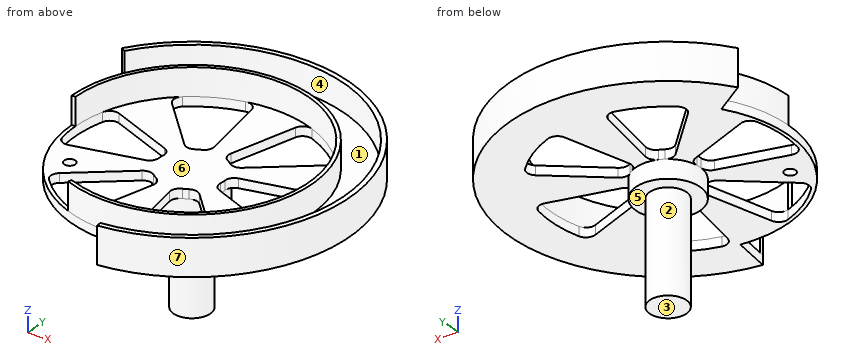
```python
from build123d import *
from build123d.topology import SkipClean

# Parameters (mm, degrees)
SCHIZZO2_R                   = 65.5
ESTRUSIONE_ESTRUSIONE1_DEPTH = 5
TAGLIO_ESTRUSIONE1_DEPTH     = 5
ESTRUSIONE_ESTRUSIONE2_START = 15
ESTRUSIONE_ESTRUSIONE2_DEPTH = 15
ESTRUSIONE_ESTRUSIONE3_DEPTH = 5
ESTRUSIONE_ESTRUSIONE4_DEPTH = 15
SCHIZZO7_R                   = 17.5
ESTRUSIONE_ESTRUSIONE5_DEPTH = 10
SCHIZZO8_R                   = 10
ESTRUSIONE_ESTRUSIONE6_DEPTH = 55
SCHIZZO9_R                   = 3
TAGLIO_ESTRUSIONE2_DEPTH     = 141.058619156


with BuildPart() as part:
    # Schizzo2 → Estrusione-Estrusione1 (new body)
    with BuildSketch(Plane.XY):
        Circle(SCHIZZO2_R)
    extrude(amount=ESTRUSIONE_ESTRUSIONE1_DEPTH)

    # Schizzo3 → Taglio-Estrusione1 (cut)
    with BuildSketch(Plane.XY.offset(5)):
        with BuildLine():
            ThreePointArc((-15.580303655, 61.558948481), (-11.6121535, 60.893291099), (-9.419229509, 57.519806288))
            Line((-9.419229509, 57.519806288), (-3.545169438, 21.649059417))
            ThreePointArc((-3.545169438, 21.649059417), (-4.118256573, 18.395634586), (-6.595126238, 16.20969802))
            ThreePointArc((-6.595126238, 16.20969802), (-7.944833745, 15.592614173), (-9.237403233, 14.863390647))
            ThreePointArc((-9.237403233, 14.863390647), (-12.461730523, 14.144422271), (-15.430658669, 15.593100175))
            Line((-15.430658669, 15.593100175), (-40.998016607, 41.429610598))
            ThreePointArc((-40.998016607, 41.429610598), (-42.438254768, 45.186607995), (-40.644362762, 48.788172498))
            ThreePointArc((-40.644362762, 48.788172498), (-28.828396733, 56.578914286), (-15.580303655, 61.558948481))
        make_face()
        with BuildLine():
            ThreePointArc((10.740447155, 13.816395873), (9.531183113, 14.676734939), (8.25337227, 15.431521188))
            ThreePointArc((8.25337227, 15.431521188), (6.018563747, 17.864386344), (5.788691541, 21.159892491))
            Line((5.788691541, 21.159892491), (15.380086943, 56.220129185))
            ThreePointArc((15.380086943, 56.220129185), (17.91362305, 59.345910719), (21.929615406, 59.593136921))
            ThreePointArc((21.929615406, 59.593136921), (34.584578723, 53.255581065), (45.521461387, 44.272413004))
            ThreePointArc((45.521461387, 44.272413004), (46.929060262, 40.503065473), (45.103998712, 36.917195183))
            Line((45.103998712, 36.917195183), (16.976050705, 13.894736502))
            ThreePointArc((16.976050705, 13.894736502), (13.871958583, 12.764332104), (10.740447155, 13.816395873))
        make_face()
        with BuildLine():
            ThreePointArc((17.335573392, -2.393302147), (17.476016858, -0.915879234), (17.490775503, 0.568130541))
            ThreePointArc((17.490775503, 0.568130541), (18.48029427, 3.719964073), (21.219350209, 5.566792317))
            Line((21.219350209, 5.566792317), (56.37810355, 14.790518587))
            ThreePointArc((56.37810355, 14.790518587), (60.351877818, 14.159302724), (62.573978168, 10.804964424))
            ThreePointArc((62.573978168, 10.804964424), (63.412975457, -3.323333221), (61.101765042, -17.286535477))
            ThreePointArc((61.101765042, -17.286535477), (58.541213762, -20.390225626), (54.523228221, -20.602611105))
            Line((54.523228221, -20.602611105), (20.521220142, -7.754322915))
            ThreePointArc((20.521220142, -7.754322915), (17.990215156, -5.631302481), (17.335573392, -2.393302147))
        make_face()
        with BuildLine():
            ThreePointArc((6.595126238, -16.20969802), (7.944833745, -15.592614173), (9.237403233, -14.863390647))
            ThreePointArc((9.237403233, -14.863390647), (12.461730523, -14.144422271), (15.430658669, -15.593100175))
            Line((15.430658669, -15.593100175), (40.998016607, -41.429610598))
            ThreePointArc((40.998016607, -41.429610598), (42.438254768, -45.186607995), (40.644362762, -48.788172498))
            ThreePointArc((40.644362762, -48.788172498), (28.828396733, -56.578914286), (15.580303655, -61.558948481))
            ThreePointArc((15.580303655, -61.558948481), (11.6121535, -60.893291099), (9.419229509, -57.519806288))
            Line((9.419229509, -57.519806288), (3.545169438, -21.649059417))
            ThreePointArc((3.545169438, -21.649059417), (4.118256573, -18.395634586), (6.595126238, -16.20969802))
        make_face()
        with BuildLine():
            ThreePointArc((-10.740447155, -13.816395873), (-9.531183113, -14.676734939), (-8.25337227, -15.431521188))
            ThreePointArc((-8.25337227, -15.431521188), (-6.018563747, -17.864386344), (-5.788691541, -21.159892491))
            Line((-5.788691541, -21.159892491), (-15.380086943, -56.220129185))
            ThreePointArc((-15.380086943, -56.220129185), (-17.91362305, -59.345910719), (-21.929615406, -59.593136921))
            ThreePointArc((-21.929615406, -59.593136921), (-34.584578723, -53.255581065), (-45.521461387, -44.272413004))
            ThreePointArc((-45.521461387, -44.272413004), (-46.929060262, -40.503065473), (-45.103998712, -36.917195183))
            Line((-45.103998712, -36.917195183), (-16.976050705, -13.894736502))
            ThreePointArc((-16.976050705, -13.894736502), (-13.871958583, -12.764332104), (-10.740447155, -13.816395873))
        make_face()
        with BuildLine():
            ThreePointArc((-17.335573392, 2.393302147), (-17.476016858, 0.915879234), (-17.490775503, -0.568130541))
            ThreePointArc((-17.490775503, -0.568130541), (-18.48029427, -3.719964073), (-21.219350209, -5.566792317))
            Line((-21.219350209, -5.566792317), (-56.37810355, -14.790518587))
            ThreePointArc((-56.37810355, -14.790518587), (-60.351877818, -14.159302724), (-62.573978168, -10.804964424))
            ThreePointArc((-62.573978168, -10.804964424), (-63.412975457, 3.323333221), (-61.101765042, 17.286535477))
            ThreePointArc((-61.101765042, 17.286535477), (-58.541213762, 20.390225626), (-54.523228221, 20.602611105))
            Line((-54.523228221, 20.602611105), (-20.521220142, 7.754322915))
            ThreePointArc((-20.521220142, 7.754322915), (-17.990215156, 5.631302481), (-17.335573392, 2.393302147))
        make_face()
    extrude(amount=-TAGLIO_ESTRUSIONE1_DEPTH, mode=Mode.SUBTRACT)

    # Schizzo4 → Estrusione-Estrusione2 (add)
    with SkipClean():  # the faces are left unmerged after this step: merging them gives an invalid solid
        with BuildSketch(Plane.XY.offset(5).offset(ESTRUSIONE_ESTRUSIONE2_START)):
            with BuildLine():
                Line((-65.499588659, 0.23213256), (-63.499601219, 0.225044543))
                ThreePointArc((-63.499601219, 0.225044543), (52.144908397, 36.23752928), (-21.929615406, -59.593136921))
                Line((-21.929615406, -59.593136921), (-22.620311954, -61.470086116))
                ThreePointArc((-22.620311954, -61.470086116), (53.787267716, 37.378868785), (-65.499588659, 0.23213256))
            make_face()
        extrude(amount=-ESTRUSIONE_ESTRUSIONE2_DEPTH)

    # Schizzo5 → Estrusione-Estrusione3 (add)
    with SkipClean():  # the faces are left unmerged after this step: merging them gives an invalid solid
        with BuildSketch(Plane.XY):
            with BuildLine():
                Line((-71.941161318, 46.719136424), (-54.9329222, 35.673856793))
                ThreePointArc((-54.9329222, 35.673856793), (55.547150298, 34.709711807), (7.982441993, -65.011772933))
                Line((7.982441993, -65.011772933), (10.453952277, -85.140608888))
                ThreePointArc((10.453952277, -85.140608888), (72.745565688, 45.456474486), (-71.941161318, 46.719136424))
            make_face()
        extrude(amount=ESTRUSIONE_ESTRUSIONE3_DEPTH)

    # Schizzo6 → Estrusione-Estrusione4 (add)
    with SkipClean():  # the faces are left unmerged after this step: merging them gives an invalid solid
        with BuildSketch(Plane.XY.offset(5)):
            with BuildLine():
                Line((-71.941161318, 46.719136424), (-69.71449096, 45.273119786))
                ThreePointArc((-69.71449096, 45.273119786), (70.493997993, 44.049538839), (10.130389171, -82.505398855))
                Line((10.130389171, -82.505398855), (10.453952277, -85.140608888))
                ThreePointArc((10.453952277, -85.140608888), (72.745565688, 45.456474486), (-71.941161318, 46.719136424))
            make_face()
        extrude(amount=ESTRUSIONE_ESTRUSIONE4_DEPTH)

    # Schizzo7 → Estrusione-Estrusione5 (add)
    with SkipClean():  # the faces are left unmerged after this step: merging them gives an invalid solid
        with BuildSketch(Plane(origin=(0, 0, 0), x_dir=(-1, 0, 0), z_dir=(0, 0, -1))):
            with Locations(Location((0, 0, 0), (0, 0, 178.139588407))):
                Circle(SCHIZZO7_R)
        extrude(amount=ESTRUSIONE_ESTRUSIONE5_DEPTH)

    # Schizzo8 → Estrusione-Estrusione6 (add)
    with SkipClean():  # the faces are left unmerged after this step: merging them gives an invalid solid
        with BuildSketch(Plane(origin=(0, 0, -10), x_dir=(-1, 0, 0), z_dir=(0, 0, -1))):
            Circle(SCHIZZO8_R)
        extrude(amount=ESTRUSIONE_ESTRUSIONE6_DEPTH)

    # Schizzo9 → Taglio-Estrusione2 (cut, through all)
    with SkipClean():  # the faces are left unmerged after this step: merging them gives an invalid solid
        with BuildSketch(Plane.XY.offset(5)):
            with Locations((-46.929060262, -26.714477403)):
                Circle(SCHIZZO9_R)
        extrude(amount=-TAGLIO_ESTRUSIONE2_DEPTH, mode=Mode.SUBTRACT)


solid = part.part
```
CAD build for the part. Positions are in the model's coordinates, mm. Face numbers are marked on the shaded views. A direction names the side the tool comes from. Round coordinates to 2 decimals unless told otherwise and drop trailing zeros. Order: outer loops, then holes, each group sorted by start corner. A loop starts at its lowest first (then second) coordinate and runs counter-clockwise, first axis right, second up.
Item 1: Saw through at B-B on y = 52.5. Write the cut outline in (x, z).
Item 2: Saw through at C-C on x = 0. Write the cut outline in (y, z) (3 decimals), then the cut area to 3 significant figures.
Item 3: Tool access for the marked faces 1, 2 and 3: list every direction of +Z, -Z, +X, -X, +Y, -Y with a clear straight run to the whole face (end or side of a thin tool).
Item 4: Pin check, flat tips, straight feed: pin 1 (5 mm diameter, centred on x = -46.93, y = -26.71, fed in from +Z); pin 2 (1.5 mm diameter, centred on y = 45, z = 0.5, fed in from -X); pin 3 (5 mm diameter, centred on x = 53.5, y = -64, fed in from -Z); pin 4 (5 mm diameter, centred on x = 41.5, z = 6.5, fed in from -Y). Stop position of each tip, or through.
Item 5: Probe line 1 along Y through (x, z) = (0, 9.5) (3 decimals); line 2 along X through (y, z) = (25, 13); line 3 along X through (y, z) = (14.5, 5.5). List the from-to ranges inside material, lowest first.
Item 6: Mould opens along X. For the marked faces 4, 5, 6 and 7 say: pulls with the +X half, pulls with the -X half, needs draft (parallel to the pull), parting line crosses it, or undercut.
Item 7: Saw through at D-D on x = 29. Write the cut outline in (y, z).
Reported:
1. outline: (-67.84, 0) - (-35.72, 0) - (-35.72, 20) - (-39.17, 20) - (-39.17, 5) - (-64.45, 5) - (-64.45, 20) - (-67.84, 20) - close; (-8.6, 0) - (14.36, 0) - (14.36, 5) - (-8.6, 5) - close; (35.72, 0) - (67.84, 0) - (67.84, 20) - (64.45, 20) - (64.45, 5) - (39.17, 5) - (39.17, 20) - (35.72, 20) - close
2. outline: (-65.5, 0) - (-17.5, 0) - (-17.5, -10) - (-10, -10) - (-10, -65) - (10, -65) - (10, -10) - (17.5, -10) - (17.5, 0) - (85.78, 0) - (85.78, 20) - (83.125, 20) - (83.125, 5) - (65.5, 5) - (65.5, 20) - (63.5, 20) - (63.5, 5) - (-63.5, 5) - (-63.5, 20) - (-65.5, 20) - close
2. area: 2,310 mm2
3. face 1: +Z
3. face 2: -Z
3. face 3: -Z, +X, -X, +Y, -Y
4. pin 1: passes through
4. pin 2: stops at x = -70.45
4. pin 3: stops at z = 0
4. pin 4: stops at y = -76.4
5. line 1: y = -65.5 to -63.5, 63.5 to 65.5, 83.125 to 85.78
5. line 2: x = -60.54 to -58.37, 58.37 to 60.54, 79.28 to 82.06
5. line 3: x = -63.87 to -61.82, 61.82 to 63.87, 81.85 to 84.55
6. face 4: undercut
6. face 5: needs draft
6. face 6: undercut
6. face 7: parting line crosses it
7. outline: (-80.73, 0) - (-56.49, 0) - (-56.49, 20) - (-58.73, 20) - (-58.73, 5) - (-77.9, 5) - (-77.9, 20) - (-80.73, 20) - close; (-29.31, 0) - (-10.96, 0) - (-10.96, 5) - (-29.31, 5) - close; (7.61, 0) - (23.74, 0) - (23.74, 5) - (7.61, 5) - close; (56.49, 0) - (80.73, 0) - (80.73, 20) - (77.9, 20) - (77.9, 5) - (58.73, 5) - (58.73, 20) - (56.49, 20) - close
